The listing builds one solid part. Answer for the finished solid, in the listing's coordinates (mm). A direction names the side the tool comes from. Give positions to 0.01 mm unless a question says otherwise; leave off trailing zeros. Order: outer loops, then holes, each group sorted by start corner. A loop starts at its lowest first (then second) coordinate and runs counter-clockwise, first axis right, second up.
```python
from build123d import *

# Parameters (mm, degrees)
SKETCH1_W                = 6
SKETCH1_H                = 6
SKETCH1_W_2              = 16
BOSS_EXTRUDE2_DEPTH      = 3
SKETCH4_W                = 5
SKETCH4_H                = 10
SKETCH4_W_2              = 10
SKETCH4_H_2              = 5
BOSS_EXTRUDE3_DEPTH      = 0.75
BOSS_EXTRUDE3_DEPTH_BACK = 0.75


with BuildPart() as part:
    # Sketch1 → Boss-Extrude2 (new body)
    with BuildSketch(Plane(origin=(0, 0, 0), x_dir=(1, 0, 0), z_dir=(0, 1, 0))):
        with Locations((0, -3)):
            Rectangle(SKETCH1_W, SKETCH1_H)
        with Locations((0, 3)):
            Rectangle(SKETCH1_W_2, SKETCH1_H)
    extrude(amount=BOSS_EXTRUDE2_DEPTH)

    # Sketch4 → Boss-Extrude3 (add, two sides)
    with BuildSketch(Plane(origin=(0, 1.5, 0), x_dir=(1, 0, 0), z_dir=(0, 1, 0))) as boss_extrude3_sk:
        with Locations((-7.5, 0)):
            Rectangle(SKETCH4_W, SKETCH4_H)
        Rectangle(SKETCH4_W_2, SKETCH4_H)
        with Locations((0, 7.5)):
            Rectangle(SKETCH4_W_2, SKETCH4_H_2)
        with Locations((7.5, 0)):
            Rectangle(SKETCH4_W, SKETCH4_H)
        with Locations((0, -7.5)):
            Rectangle(SKETCH4_W_2, SKETCH4_H_2)
    extrude(amount=BOSS_EXTRUDE3_DEPTH)
    extrude(boss_extrude3_sk.sketch, amount=-BOSS_EXTRUDE3_DEPTH_BACK)


solid = part.part
```
1) Find section B-B (y = 1.5). Write down the section's boundary in (x, z).
Geometry says:
outline: (-10, -5) - (-8, -5) - (-8, -6) - (-5, -6) - (-5, -10) - (5, -10) - (5, -6) - (8, -6) - (8, -5) - (10, -5) - (10, 5) - (5, 5) - (5, 10) - (-5, 10) - (-5, 5) - (-10, 5) - close
2) Find section D-D (y = 0.3). Write down the section's boundary in (x, z).
Geometry says:
outline: (-8, -6) - (8, -6) - (8, 0) - (3, 0) - (3, 6) - (-3, 6) - (-3, 0) - (-8, 0) - close
3) A tool of negligible diameter and unlimited length cuts with its end or side. For faces 1 (the flat face through (0, 0.75, -8)), 2 (the flat face through (7, 2, 5)), 3 (the flat face through (-8, 2, 5)), 4 (the flat face through (5, 1, -8)), from which of +Z, -Z, +X, -X, +Y, -Y can it reach the whole face along a straight path? Write none if from no direction.
Geometry says:
face 1: -Z, +X, -X, -Y
face 2: +Z, +X, +Y, -Y
face 3: +Z, -X, +Y, -Y
face 4: -Z, +X, +Y, -Y
4) Find section C-C (z = 5.75). Write down the section's boundary in (x, y).
Geometry says:
outline: (-5, 0.75) - (-3, 0.75) - (-3, 0) - (3, 0) - (3, 0.75) - (5, 0.75) - (5, 2.25) - (3, 2.25) - (3, 3) - (-3, 3) - (-3, 2.25) - (-5, 2.25) - close
5) Straight lines are drawn through the part: probe 1 along Z at (x, y) = (2, 2.7); probe 2 along Z at (x, y) = (-6.5, 0.45); probe 3 along X at (y, z) = (1.25, 5.5). For each, find the intervals that lie inside material, in ascending order.
Geometry says:
probe 1: z = -6 to 6
probe 2: z = -6 to 0
probe 3: x = -5 to 5
6) Find section A-A (x = -0.5). Write down the section's boundary in (y, z), then the cut area to 3 significant figures.
Geometry says:
outline: (0, -6) - (0.75, -6) - (0.75, -10) - (2.25, -10) - (2.25, -6) - (3, -6) - (3, 6) - (2.25, 6) - (2.25, 10) - (0.75, 10) - (0.75, 6) - (0, 6) - close
area: 48.0 mm2
7) Given P1, Ø0.6, axis at x = 4.5, y = 2.5, coming from the +Z side; P2, Ø0.8, axis at y = 1.5, z = 6.5, coming from the +X side; P3, Ø1.6, axis at x = 6.5, y = 2, coming from the +Z side; P4, Ø1.5, axis at x = 0.5, z = 8, coming from the -Y side, each flat-ended and moving along its own axis, determine where each tip first touches the part or whether it passes through.
Geometry says:
P1: stops at z = 10
P2: stops at x = 5
P3: stops at z = 5
P4: stops at y = 0.75
